Verification items for the finished model (mm, model axes). A direction names the side the tool comes from. Give positions to 0.01 mm unless a question says otherwise; leave off trailing zeros. Order: outer loops, then holes, each group sorted by start corner. A loop starts at its lowest first (then second) coordinate and runs counter-clockwise, first axis right, second up. Notation, with made-up numbers: (21, 62) -> (26, 62) arc R25 cw to (26, 100) -> close; hole circle Ø4 at (13, 9). An arc over 180 degrees is marked (long way). One line per question, with ' | ' between items. Start each with the question number.
Q1. Mould release check, pull along Z, two halves, no side actions. Record for faces 5 (the flat face through (243.423, -9, 513)), 6 (the flat face through (12, -11, 208.201)), 7 (the flat face through (18, -9, 538.401)), 8 (the flat face through (12, -11, 81.201)): released by +Z, released by -Z, zero draft, split by the parting line, or undercut.
Q2. Access from +Z, -Z, +X, -X, +Y, -Y to the whole of each face (thin tool, end or side, straight path). Record for faces 1 (the flat face through (-213.777, -9, 513)), 2 (the flat face through (12, -11, 220.901)), 3 (the flat face through (-188.377, -1, 212)), 4 (the flat face through (218.023, -9, 266)).
Q3. Section check A-A on y = -9.75. Give the number of separate pieces and of enclosed holes in the cut face, plus the area to 3 significant figures.
Q4. Go/stop test with flat-tipped pins: pin 1 (3 mm diameter, centred on x = -71, z = 45.5, fed in from -Y); pin 2 (10 mm diameter, centred on y = -17, z = 180, fed in from +X); pin 3 (9.5 mm diameter, centred on y = -6, z = 124, fed in from -X). Record where each tip stops, or that it passes through.
Q5. Section check B-B on z = 269. Record the cut outline in (x, y), plus the area to 3 significant figures.
Q6. Material ranges on probe 1 along X at (y, z) = (-14.5, -35.5); probe 2 along Z at (x, y) = (222.5, -0.75); probe 3 along Z at (x, y) = (-154, -2.25), recorded low to high. Write a range as [from, to].
from build123d import *

# Parameters (mm, degrees)
F1_DEPTH = 19.05
F2_W     = 406.4
F2_H     = 6.35
F3_DEPTH = 16.51
F4_W     = 406.4
F4_H     = 31.75
F5_DEPTH = 12.7


with BuildPart() as f1:
    # F0 (on Front) → F1 (new body)
    with BuildSketch(Plane.XZ):
        Polygon((218.022645, -71.199347), (218.022645, 487.600653), (243.422645, 487.600653), (243.422645, 538.400653), (-213.777355, 538.400653), (-213.777355, 487.600653), (-188.377355, 487.600653), (-188.377355, -71.199347), align=None)
    extrude(amount=F1_DEPTH)

    # F2 (on face) → F3 (cut)
    with BuildSketch(Plane.XZ.offset(19.05)):
        with Locations((14.822645, -17.224347)):
            Rectangle(F2_W, F2_H)
        with Locations((14.822645, -4.524347)):
            Rectangle(F2_W, F2_H)
        with Locations((14.822645, 8.175653)):
            Rectangle(F2_W, F2_H)
        with Locations((14.822645, 20.875653)):
            Rectangle(F2_W, F2_H)
        with Locations((14.822645, 33.575653)):
            Rectangle(F2_W, F2_H)
        with Locations((14.822645, 46.275653)):
            Rectangle(F2_W, F2_H)
        with Locations((14.822645, 58.975653)):
            Rectangle(F2_W, F2_H)
        with Locations((14.822645, 71.675653)):
            Rectangle(F2_W, F2_H)
        with Locations((14.822645, 84.375653)):
            Rectangle(F2_W, F2_H)
        with Locations((14.822645, 97.075653)):
            Rectangle(F2_W, F2_H)
        with Locations((14.822645, 109.775653)):
            Rectangle(F2_W, F2_H)
        with Locations((14.822645, 122.475653)):
            Rectangle(F2_W, F2_H)
        with Locations((14.822645, 135.175653)):
            Rectangle(F2_W, F2_H)
        with Locations((14.822645, 147.875653)):
            Rectangle(F2_W, F2_H)
        with Locations((14.822645, 160.575653)):
            Rectangle(F2_W, F2_H)
        with Locations((14.822645, 173.275653)):
            Rectangle(F2_W, F2_H)
        with Locations((14.822645, 185.975653)):
            Rectangle(F2_W, F2_H)
        with Locations((14.822645, 198.675653)):
            Rectangle(F2_W, F2_H)
        with Locations((14.822645, 211.375653)):
            Rectangle(F2_W, F2_H)
        with Locations((14.822645, 224.075653)):
            Rectangle(F2_W, F2_H)
        with Locations((14.822645, 236.775653)):
            Rectangle(F2_W, F2_H)
        with Locations((14.822645, 249.475653)):
            Rectangle(F2_W, F2_H)
    extrude(amount=-F3_DEPTH, mode=Mode.SUBTRACT)

    # F4 (on face) → F5 (cut)
    with BuildSketch(Plane(origin=(0, 0, 0), x_dir=(-1, 0, 0), z_dir=(0, 1, 0))):
        with Locations((-14.822645, -55.324347)):
            Rectangle(F4_W, F4_H)
    extrude(amount=-F5_DEPTH, mode=Mode.SUBTRACT)


solid = f1.part
Filled in:
1) face 5: zero draft | face 6: undercut | face 7: released by +Z | face 8: undercut
2) face 1: +Z, -Z, -X, +Y, -Y | face 2: +X, -X, -Y | face 3: -Z, -X, +Y, -Y | face 4: -Z, +X, +Y, -Y
3) separate pieces: 23 | enclosed holes: 0 | area: 181,000 mm²
4) pin 1: y = -2.54 | pin 2: x = 218.02 | pin 3: x = -188.38
5) outline: (-188.38, -19.05) -> (218.02, -19.05) -> (218.02, 0) -> (-188.38, 0) -> close | area: 7,740 mm²
6) probe 1: [-188.38, 218.02] | probe 2: [487.6, 538.4] | probe 3: [-39.45, 538.4]
